from build123d import *

# Parameters (mm, degrees)
F0_W     = 60
F0_H     = 60
F1_DEPTH = 10
F2_R     = 10
F3_R     = 16
F4_DEPTH = 30
F6_D     = 14
F8_D     = 10


with BuildPart() as f1:
    # F0 (on Front) → F1 (new body)
    with BuildSketch(Plane.XZ):
        Rectangle(F0_W, F0_H)
    extrude(amount=F1_DEPTH)

    # F2
    f2_edges = [f1.edges().sort_by_distance(p)[0] for p in [
        (30, -5, 30),
        (-30, -5, 30),
        (30, -5, -30),
        (-30, -5, -30),
    ]]
    fillet(f2_edges, radius=F2_R)

    # F3 (on face) → F4 (join)
    with BuildSketch(Plane.XZ.offset(10)):
        Circle(F3_R)
    extrude(amount=F4_DEPTH)

    # F6 (through all)
    with Locations(Plane.XZ.offset(40)):
        with Locations((0, 0)):
            Hole(F6_D / 2)

    # F8 (through all)
    with Locations(Plane.XZ.offset(40)):
        with Locations((-20, 20), (20, 20), (20, -20), (-20, -20)):
            Hole(F8_D / 2)


solid = f1.part
Could you check a few things on this model? Use its own coordinates, in mm. A direction names the side the tool comes from. Coordinates: 2 decimals unless noted, no trailing zeros. Write each loop counter-clockwise with the first axis right and the second up, starting at its lowest first coordinate (ties: lowest second). Pieces come first, ordered by that corner, then holes. Notation, with made-up numbers: (73.25, 88.5) - (110.25, 88.5) arc R23 ccw to (110.25, 122.5) - close; hole circle Ø4 at (70.25, -23). An arc over 180 degrees is marked (long way). Write item = value, one per line.
1) For faces 1 (the flat face through (13, -10, -13)), 2 (the cylindrical face through (27.15, -5.07, 26.99)), which set-ups out of +Z, -Z, +X, -X, +Y, -Y let a thin tool reach every point of the face, with its end or its side?
Result set:
face_1 = -Y
face_2 = +Z, +X, +Y, -Y
2) Suppose I cut it at A-A on x = 0. Please give me the cut outline in (y, z), plus the area to 3 significant figures.
Result set:
outline = (-40, -16) - (-10, -16) - (-10, -30) - (0, -30) - (0, -7) - (-40, -7) - close; (-40, 7) - (0, 7) - (0, 30) - (-10, 30) - (-10, 16) - (-40, 16) - close
area = 1,000 mm2
3) Suppose I cut it at B-B on y = -8. Please give me the cut outline in (x, z), plus the area to 3 significant figures.
Result set:
outline = (-30, -20) arc R10 ccw to (-20, -30) - (20, -30) arc R10 ccw to (30, -20) - (30, 20) arc R10 ccw to (20, 30) - (-20, 30) arc R10 ccw to (-30, 20) - close; hole circle Ø10 at (-20, -20); hole circle Ø10 at (-20, 20); hole circle Ø14 at (0, 0); hole circle Ø10 at (20, -20); hole circle Ø10 at (20, 20)
area = 3,050 mm2
4) Suppose I cut it at D-D on z = 0. Please give me the cut outline in (x, y), plus the area to 3 significant figures.
Result set:
outline = (-30, -10) - (-16, -10) - (-16, -40) - (-7, -40) - (-7, 0) - (-30, 0) - close; (7, -40) - (16, -40) - (16, -10) - (30, -10) - (30, 0) - (7, 0) - close
area = 1,000 mm2
5) We'd pull the mould along Z, two halves only. Please class faces 3 (the cylindrical face through (-18.92, -4.93, -24.88)), 4 (the cylindrical face through (-3.47, -24.79, -15.62)), 5 (the flat face through (7, -40, -3)), 6 (the cylindrical face through (21.08, -4.93, -24.88)): +Z half, -Z half, draft (parallel to the pull), parting line (faces both ways), or undercut.
Result set:
face_3 = undercut
face_4 = parting line
face_5 = draft
face_6 = undercut
6) Will these pins go through, and if not, where does the flat tip stop? pin 1 Ø12.5 at (x, z) = (0, 0) entering from -Y; pin 2 Ø5 at (y, z) = (-20, 7) entering from +X; pin 3 Ø16 at (x, z) = (-20, -20) entering from -Y; pin 4 Ø1.5 at (x, y) = (-14.5, -19) entering from +Z.
Result set:
pin_1 = through
pin_2 = 15.35
pin_3 = -10
pin_4 = 8.18
7) Please list where these lines run through material, in increasing order: line 1 (Z direction, x = 20, y = -6); line 2 (X direction, y = -3.5, z = 19); line 3 (Z direction, x = 0, y = -21.5). Write a range as [from, to].
Result set:
line_1 = [-30, -25], [-15, 15], [25, 30]
line_2 = [-30, -24.9], [-15.1, 15.1], [24.9, 30]
line_3 = [-16, -7], [7, 16]
8) Suppose I cut it at C-C on z = -17. Please give me the cut outline in (x, y).
Result set:
outline = (-30, -10) - (-24, -10) - (-24, 0) - (-30, 0) - close; (-16, -10) - (16, -10) - (16, 0) - (-16, 0) - close; (24, -10) - (30, -10) - (30, 0) - (24, 0) - close
